from build123d import *

# Parameters (mm, degrees)
F1_DEPTH = 44
F2_W     = 25
F2_H     = 12
F3_DEPTH = 12
F4_W     = 25
F4_H     = 12
F5_DEPTH = 12


with BuildPart() as f1:
    # F0 (on Front) → F1 (new body)
    with BuildSketch(Plane.XZ):
        Polygon((-35, 7.5), (-15, -32.5), (15, -32.5), (35, 7.5), (35, 32.5), (-35, 32.5), align=None)
    extrude(amount=F1_DEPTH)

    # F2 (on face) → F3 (join)
    with BuildSketch(Plane(origin=(-35, 0, 0), x_dir=(0, -1, 0), z_dir=(-1, 0, 0))):
        with Locations((31.5, 26.5)):
            Rectangle(F2_W, F2_H)
    extrude(amount=F3_DEPTH)

    # F4 (on face) → F5 (join)
    with BuildSketch(Plane.YZ.offset(35)):
        with Locations((-31.5, 26.5)):
            Rectangle(F4_W, F4_H)
    extrude(amount=F5_DEPTH)


solid = f1.part
Design review of the part built by this model. Coordinates are the model's own, in mm. A direction names the side the tool comes from. Round coordinates to 2 decimals unless told otherwise and drop trailing zeros. Order: outer loops, then holes, each group sorted by start corner. A loop starts at its lowest first (then second) coordinate and runs counter-clockwise, first axis right, second up.
1) Consider section B-B (z = 23.5). State the section outline as (x, y) points.
The answers:
outline: (-47, -44) - (47, -44) - (47, -19) - (35, -19) - (35, 0) - (-35, 0) - (-35, -19) - (-47, -19) - close
2) Clearance check with flat-ended pins moving along their axes: pin 1 Ø2 at (y, z) = (-29.5, -14) entering from -X; pin 2 Ø5 at (y, z) = (-39.5, -23) entering from -X; pin 3 Ø1.5 at (y, z) = (-16, 7.5) entering from -X. State where each tip first meets the part, or that it passes through.
The answers:
pin 1: stops at x = -24.75
pin 2: stops at x = -21
pin 3: stops at x = -35
3) Consider section D-D (y = -16.5). State the section outline as (x, z) points.
The answers:
outline: (-35, 7.5) - (-15, -32.5) - (15, -32.5) - (35, 7.5) - (35, 32.5) - (-35, 32.5) - close
4) Consider section C-C (x = 39.5). State the section outline as (y, z) points, plus the area to 3 significant figures.
The answers:
outline: (-44, 20.5) - (-19, 20.5) - (-19, 32.5) - (-44, 32.5) - close
area: 300 mm2
5) Machinability: for faces 1 (the flat face through (41, -19, 26)), 2 (the flat face through (-41, -19, 26)), 3 (the flat face through (-41, -31, 20.5)), 4 (the flat face through (41, -32, 20.5)), which of the approach directions +Z, -Z, +X, -X, +Y, -Y give a long, thin tool a straight path to every point of the face, cutting with its end or side? Answer none if there is none.
The answers:
face 1: +Z, -Z, +X, +Y
face 2: +Z, -Z, -X, +Y
face 3: -Z, -X, +Y, -Y
face 4: -Z, +X, +Y, -Y
6) Consider section A-A (y = -34.5). State the section outline as (x, z) points.
The answers:
outline: (-47, 20.5) - (-35, 20.5) - (-35, 7.5) - (-15, -32.5) - (15, -32.5) - (35, 7.5) - (35, 20.5) - (47, 20.5) - (47, 32.5) - (-47, 32.5) - close
7) For L1, parallel to X at y = -18, z = 12; L2, parallel to Z at x = -38, y = -32; L3, parallel to X at y = -22, z = -26.5, list the stretches that pass through material, from the lowest coordinate up.
The answers:
L1: x = -35 to 35
L2: z = 20.5 to 32.5
L3: x = -18 to 18
